Work out the finished part from the listing and answer in its coordinate system (mm). A direction names the side the tool comes from. Coordinates: 2 decimals unless noted, no trailing zeros. Order: outer loops, then holes, each group sorted by start corner. A loop starts at its lowest first (then second) coordinate and runs counter-clockwise, first axis right, second up. Notation, with made-up numbers: M 16.25,23.5 L 67.25,23.5 A16 ccw 67.25,29.5 Z; hole C -32.5,-16.5 d7. An arc over 180 degrees is marked long. Use a Markdown table: item, result.
Autodesk Inventor part; units mm, degrees
ref_plane "YZ Plane" through (0, 0, 0) normal (1, 0, 0) x (0, 1, 0)
ref_plane "XZ Plane" through (0, 0, 0) normal (0, 1, 0) x (-1, 0, 0)
ref_plane "XY Plane" through (0, 0, 0) normal (0, 0, 1) x (1, 0, 0)
sketch "Эскиз1" plane through (0, 0, 0) normal (1, 0, 0) x (0, 1, 0)
  line L0 (152.4218, -265.1334) -> (152.4218, -277.6334)
  line L1 (152.4218, -277.6334) -> (177.4218, -277.6334)
  line L2 (177.4218, -277.6334) -> (177.4218, -269.6855)
  line L3 (176.5549, -268.0374) -> (169.9337, -263.4853)
  line L4 (154.4218, -263.1334) -> (168.8006, -263.1334)
  line L5 (153.4218, -267.6334) -> (157.9218, -267.6334)
  line L6 (157.9218, -267.6334) -> (157.9218, -272.1334)
  line L7 (157.9218, -272.1334) -> (153.4218, -272.1334)
  line L8 (153.4218, -272.1334) -> (153.4218, -267.6334)
  line L9 (177.4218, -277.6334) -> (177.4218, -269.6855)
  line L10 (176.5549, -268.0374) -> (169.9337, -263.4853)
  circle A0 centre (163.9218, -266.1334) radius 2
  circle A1 centre (172.9218, -271.1334) radius 2
  arc A2 (154.4218, -263.1334) -> (152.4218, -265.1334) centre (154.4218, -265.1334) ccw
  arc A3 (169.9337, -263.4853) -> (168.8006, -263.1334) centre (168.8006, -265.1334) ccw
  arc A4 (177.4218, -269.6855) -> (176.5549, -268.0374) centre (175.4218, -269.6855) ccw
  line L11 (152.4218, -290.1334) -> (152.4218, -277.6334)
  line L12 (177.4218, -277.6334) -> (177.4218, -285.5814)
  line L13 (176.5549, -287.2295) -> (169.9337, -291.7815)
  circle A5 centre (172.9218, -284.1334) radius 2
  circle A6 centre (163.9218, -289.1334) radius 2
  line L14 (157.9218, -287.6334) -> (157.9218, -283.1334)
  line L15 (157.9218, -283.1334) -> (153.4218, -283.1334)
  line L16 (153.4218, -283.1334) -> (153.4218, -287.6334)
  line L17 (154.4218, -292.1334) -> (168.8006, -292.1334)
  line L18 (153.4218, -287.6334) -> (157.9218, -287.6334)
  arc A7 (152.4218, -290.1334) -> (154.4218, -292.1334) centre (154.4218, -290.1334) ccw
  arc A8 (168.8006, -292.1334) -> (169.9337, -291.7815) centre (168.8006, -290.1334) ccw
  arc A9 (176.5549, -287.2295) -> (177.4218, -285.5814) centre (175.4218, -285.5814) ccw
  dimension "d181" = 5.5
  dimension "d182" = 1
  dimension "d183" = 4.5
  dimension "d184" = 4.5
  dimension "d185" = 6
  dimension "d186" = 5
  dimension "d187" = 3
  dimension "d188" = 9
extrude "Выдавливание3" add sketch "Эскиз1" along normal blind 2
properties part number "Практика галактика"
1. A flat-ended cylindrical pin translates along its axis: P1, Ø0.6, axis at x = 1, z = -286, coming from the +Y side. Find the tip coordinate at first contact, or state that the pin passes through.
Answers below:
| item | result |
|---|---|
| P1 | y = 177.42 |
2. Section C-C on y = 174.5 is taken. Determine the outline of the cut face in (x, z), then the cut area to 3 significant figures.
Answers below:
| item | result |
|---|---|
| outline | M 0,-288.64 L 2,-288.64 L 2,-285.36 L 0,-285.36 Z; M 0,-282.9 L 2,-282.9 L 2,-272.36 L 0,-272.36 Z; M 0,-269.9 L 2,-269.9 L 2,-266.62 L 0,-266.62 Z |
| area | 34.2 mm² |
3. For faces 4 (the face through (1, 156, -283.133)), 5 (the face through (0, 165, -277)), determine the directions among +Z, -Z, +X, -X, +Y, -Y from which every point of the face is accessible in a straight line to the end or side of a thin tool.
Answers below:
| item | result |
|---|---|
| face 4 | +X, -X |
| face 5 | +Z, -Z, -X, +Y, -Y |
4. Find the intervals of material crossed by probe 1 along Z at (x, y) = (1.55, 157.5); probe 2 along Y at (x, z) = (1.65, -284); probe 3 along Z at (x, y) = (1.25, 172.5), in increasing order.
Answers below:
| item | result |
|---|---|
| probe 1 | -292.13 to -287.63, -283.13 to -272.13, -267.63 to -263.13 |
| probe 2 | 152.42 to 153.42, 157.92 to 170.93, 174.92 to 177.42 |
| probe 3 | -290.02 to -286.09, -282.18 to -273.09, -269.18 to -265.25 |
5. For a pull along Z with two mould halves and no side action, classify faces 1 (the face through (0.986, 169.386, -263.221)), 2 (the face through (0.99, 169.4, -292.04)), 3 (the face through (1, 156, -267.633)) as +Z half, -Z half, draft (parallel to the pull), parting line (faces both ways), or undercut.
Answers below:
| item | result |
|---|---|
| face 1 | +Z half |
| face 2 | -Z half |
| face 3 | undercut |
6. Section B-B on x = 0.45 is taken. Determine the outline of the cut face in (y, z), then the cut area to 3 significant figures.
Answers below:
| item | result |
|---|---|
| outline | M 152.42,-290.13 A2 ccw 154.42,-292.13 L 168.8,-292.13 A2 ccw 169.93,-291.78 L 176.55,-287.23 A2 ccw 177.42,-285.58 L 177.42,-269.69 A2 ccw 176.55,-268.04 L 169.93,-263.49 A2 ccw 168.8,-263.13 L 154.42,-263.13 A2 ccw 152.42,-265.13 Z; hole M 153.42,-287.63 L 157.92,-287.63 L 157.92,-283.13 L 153.42,-283.13 Z; hole M 153.42,-272.13 L 157.92,-272.13 L 157.92,-267.63 L 153.42,-267.63 Z; hole C 163.92,-289.13 d4; hole C 163.92,-266.13 d4; hole C 172.92,-284.13 d4; hole C 172.92,-271.13 d4 |
| area | 588 mm² |
7. Section A-A on y = 164.75 is taken. Determine the outline of the cut face in (x, z).
Answers below:
| item | result |
|---|---|
| outline | M 0,-292.13 L 2,-292.13 L 2,-290.95 L 0,-290.95 Z; M 0,-287.31 L 2,-287.31 L 2,-267.95 L 0,-267.95 Z; M 0,-264.31 L 2,-264.31 L 2,-263.13 L 0,-263.13 Z |
